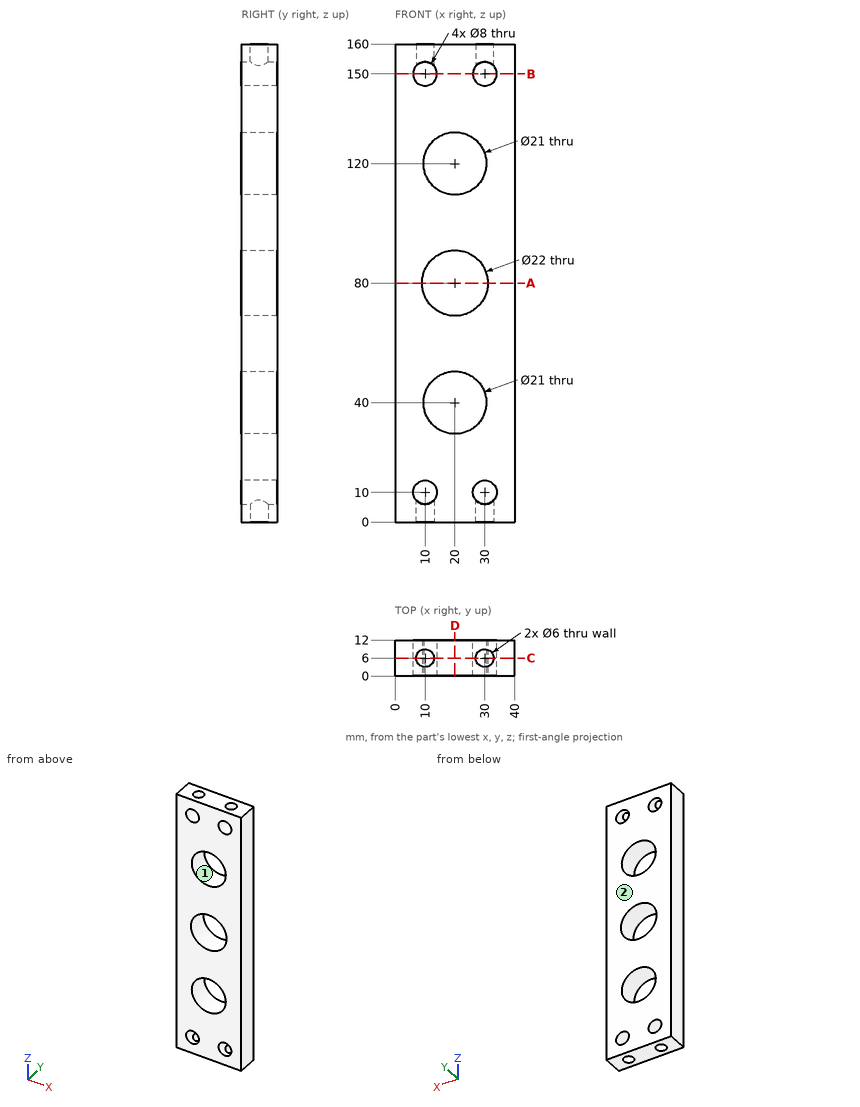
The figure shows three views and two pictorial views of one solid part (mm, origin at its lowest corner). Answer the questions. Coordinates: 2 decimals unless noted, no trailing zeros. Write each loop counter-clockwise with the first axis right and the second up, starting at its lowest first coordinate (ties: lowest second). Pieces come first, ordered by that corner, then holes. Notation, with made-up numbers: (57, 61.5) -> (84, 61.5) arc R16 cw to (84, 77.5) -> close; hole circle Ø3 at (84, 2). An arc over 180 degrees is marked (long way). Return JSON: item names as keys, results as strings.
(1) For a pull along Z with two mould halves and no side action, classify the marked faces 1 and 2 as pulls with the +Z half, pulls with the -Z half, needs draft (parallel to the pull), parting line crosses it, or undercut.
Answers below:
{"face 1": "undercut", "face 2": "needs draft"}
(2) The part is cut by section D-D on x = 20. Give the vertices of the cut face in (y, z), then the cut area to 3 significant figures.
Answers below:
{"outline": "(0, 0) -> (12, 0) -> (12, 29.5) -> (0, 29.5) -> close; (0, 50.5) -> (12, 50.5) -> (12, 69) -> (0, 69) -> close; (0, 91) -> (12, 91) -> (12, 109.5) -> (0, 109.5) -> close; (0, 130.5) -> (12, 130.5) -> (12, 160) -> (0, 160) -> close", "area": "1,150 mm^2"}
(3) Each of these flat-tipped pins is pushed along its axis until it touches: P1, Ø17, axis at x = 20, z = 40, coming from the -Y side; P2, Ø6, axis at y = 6.5, z = 124, coming from the -X side; P3, Ø5.5, axis at x = 10, y = 6, coming from the +Z side. Where does it stop, or does it pass through?
Answers below:
{"P1": "through", "P2": "x = 0", "P3": "z = 147.1"}
(4) The part is cut by section B-B on z = 150. Give the vertices of the cut face in (x, y).
Answers below:
{"outline": "(0, 0) -> (6, 0) -> (6, 12) -> (0, 12) -> close; (14, 0) -> (26, 0) -> (26, 12) -> (14, 12) -> close; (34, 0) -> (40, 0) -> (40, 12) -> (34, 12) -> close"}
(5) The part is cut by section C-C on y = 6. Give the vertices of the cut face in (x, z), then the cut area to 3 significant figures.
Answers below:
{"outline": "(0, 0) -> (7, 0) -> (7, 7.35) arc R4 cw (long way) to (13, 7.35) -> (13, 0) -> (27, 0) -> (27, 7.35) arc R4 cw (long way) to (33, 7.35) -> (33, 0) -> (40, 0) -> (40, 160) -> (33, 160) -> (33, 152.65) arc R4 cw (long way) to (27, 152.65) -> (27, 160) -> (13, 160) -> (13, 152.65) arc R4 cw (long way) to (7, 152.65) -> (7, 160) -> (0, 160) -> close; hole circle Ø22 at (20, 80); hole circle Ø21 at (20, 40); hole circle Ø21 at (20, 120)", "area": "4,970 mm^2"}
(6) Consider line 1 along Z through (x, y) = (20.5, 10.5); line 2 along Y through (x, z) = (10, 154.75); line 3 along Z through (x, y) = (6.5, 9.25). Determine where each line is inside the solid, lowest interval first. Write a range as from..to.
Answers below:
{"line 1": "0..29.51, 50.49..69.01, 90.99..109.51, 130.49..160", "line 2": "0..3, 9..12", "line 3": "0..8.06, 11.94..148.06, 151.94..160"}
(7) The part is cut by section A-A on z = 80. Give the vertices of the cut face in (x, y).
Answers below:
{"outline": "(0, 0) -> (9, 0) -> (9, 12) -> (0, 12) -> close; (31, 0) -> (40, 0) -> (40, 12) -> (31, 12) -> close"}
